from build123d import *

# Parameters (mm, degrees)
F0_R           = 29
F1_DEPTH       = 6
F9_R           = 1.5
F12_DEPTH      = 5
F12_DEPTH_BACK = 10
F10_R          = 1.5
F13_DEPTH      = 5
F13_DEPTH_BACK = 10
F8_R           = 1.5
F14_DEPTH      = 5
F14_DEPTH_BACK = 10
F11_R          = 1.5
F15_DEPTH      = 5
F15_DEPTH_BACK = 10
F4_R           = 1.5
F16_DEPTH      = 5
F16_DEPTH_BACK = 10
F7_R           = 1.5
F17_DEPTH      = 5
F17_DEPTH_BACK = 10
F6_R           = 1.5
F18_DEPTH      = 5
F18_DEPTH_BACK = 10
F5_R           = 1.5
F19_DEPTH      = 5
F19_DEPTH_BACK = 10
F3_R           = 1.5
F20_DEPTH      = 5
F20_DEPTH_BACK = 10
F21_R          = 36.5
F21_R_2        = 31.775
F22_DEPTH      = 6
F2_R           = 1.5
F23_DEPTH      = 10


with BuildPart() as f1:
    # F0 (on Top) → F1 (new body)
    with BuildSketch(Plane.XY):
        Polygon((33.286979, -10.815593), (33.286977, 10.815597), (20.572482, 28.315596), (-2e-06, 35), (-20.572485, 28.315594), (-33.286979, 10.815593), (-33.286977, -10.815597), (-20.572482, -28.315596), (2e-06, -35), (20.572485, -28.315594), align=None)
        Circle(F0_R, mode=Mode.SUBTRACT)
    extrude(amount=F1_DEPTH)

    # F9 (on face) → F12 (cut, two sides)
    with BuildSketch(Plane(origin=(-33.286978, -2e-06, 0), x_dir=(0, -1, 0), z_dir=(-1, 0, 0))) as f12_sk:
        with Locations((0.000595, 3)):
            Circle(F9_R)
    extrude(amount=-F12_DEPTH, mode=Mode.SUBTRACT)
    extrude(f12_sk.sketch, amount=-F12_DEPTH_BACK, mode=Mode.SUBTRACT)

    # F10 (on face) → F13 (cut, two sides)
    with BuildSketch(Plane(origin=(10.286244, -31.657797, 0), x_dir=(0.951056, 0.309017, 0), z_dir=(0.309017, -0.951056, 0))) as f13_sk:
        with Locations((-1.499405, 3)):
            Circle(F10_R)
    extrude(amount=-F13_DEPTH, mode=Mode.SUBTRACT)
    extrude(f13_sk.sketch, amount=-F13_DEPTH_BACK, mode=Mode.SUBTRACT)

    # F8 (on face) → F14 (cut, two sides)
    with BuildSketch(Plane(origin=(33.286978, 2e-06, 0), x_dir=(0, 1, 0), z_dir=(1, 0, 0))) as f14_sk:
        with Locations((0.000595, 3)):
            Circle(F8_R)
    extrude(amount=F14_DEPTH, mode=Mode.SUBTRACT)
    extrude(f14_sk.sketch, amount=-F14_DEPTH_BACK, mode=Mode.SUBTRACT)

    # F11 (on face) → F15 (cut, two sides)
    with BuildSketch(Plane(origin=(26.929732, -19.565593, 0), x_dir=(0.587785, 0.809017, 0), z_dir=(0.809017, -0.587785, 0))) as f15_sk:
        with Locations((-1.499405, 3)):
            Circle(F11_R)
    extrude(amount=F15_DEPTH, mode=Mode.SUBTRACT)
    extrude(f15_sk.sketch, amount=-F15_DEPTH_BACK, mode=Mode.SUBTRACT)

    # F4 (on face) → F16 (cut, two sides)
    with BuildSketch(Plane(origin=(-26.92973, -19.565596, 0), x_dir=(0.587785, -0.809017, 0), z_dir=(-0.809017, -0.587785, 0))) as f16_sk:
        with Locations((0.000595, 3)):
            Circle(F4_R)
    extrude(amount=F16_DEPTH, mode=Mode.SUBTRACT)
    extrude(f16_sk.sketch, amount=-F16_DEPTH_BACK, mode=Mode.SUBTRACT)

    # F7 (on face) → F17 (cut, two sides)
    with BuildSketch(Plane(origin=(-26.929732, 19.565593, 0), x_dir=(-0.587785, -0.809017, 0), z_dir=(-0.809017, 0.587785, 0))) as f17_sk:
        with Locations((0.000595, 3)):
            Circle(F7_R)
    extrude(amount=F17_DEPTH, mode=Mode.SUBTRACT)
    extrude(f17_sk.sketch, amount=-F17_DEPTH_BACK, mode=Mode.SUBTRACT)

    # F6 (on face) → F18 (cut, two sides)
    with BuildSketch(Plane(origin=(26.92973, 19.565596, 0), x_dir=(-0.587785, 0.809017, 0), z_dir=(0.809017, 0.587785, 0))) as f18_sk:
        with Locations((0.000595, 3)):
            Circle(F6_R)
    extrude(amount=-F18_DEPTH, mode=Mode.SUBTRACT)
    extrude(f18_sk.sketch, amount=-F18_DEPTH_BACK, mode=Mode.SUBTRACT)

    # F5 (on face) → F19 (cut, two sides)
    with BuildSketch(Plane(origin=(-10.28624, -31.657798, 0), x_dir=(0.951057, -0.309017, 0), z_dir=(-0.309017, -0.951057, 0))) as f19_sk:
        with Locations((0.000595, 3)):
            Circle(F5_R)
    extrude(amount=-F19_DEPTH, mode=Mode.SUBTRACT)
    extrude(f19_sk.sketch, amount=-F19_DEPTH_BACK, mode=Mode.SUBTRACT)

    # F3 (on face) → F20 (cut, two sides)
    with BuildSketch(Plane(origin=(10.28624, 31.657798, 0), x_dir=(-0.951057, 0.309017, 0), z_dir=(0.309017, 0.951057, 0))) as f20_sk:
        with Locations((0.000595, 3)):
            Circle(F3_R)
    extrude(amount=-F20_DEPTH, mode=Mode.SUBTRACT)
    extrude(f20_sk.sketch, amount=-F20_DEPTH_BACK, mode=Mode.SUBTRACT)

    # F21 (on Top) → F22 (cut)
    with BuildSketch(Plane.XY):
        Circle(F21_R)
        Circle(F21_R_2, mode=Mode.SUBTRACT)
    extrude(amount=F22_DEPTH, mode=Mode.SUBTRACT)

    # F2 (on face) → F23 (cut)
    with BuildSketch(Plane(origin=(-10.286244, 31.657797, 0), x_dir=(-0.951056, -0.309017, 0), z_dir=(-0.309017, 0.951056, 0))):
        with Locations((0.000595, 3)):
            Circle(F2_R)
    extrude(amount=-F23_DEPTH, mode=Mode.SUBTRACT)


solid = f1.part
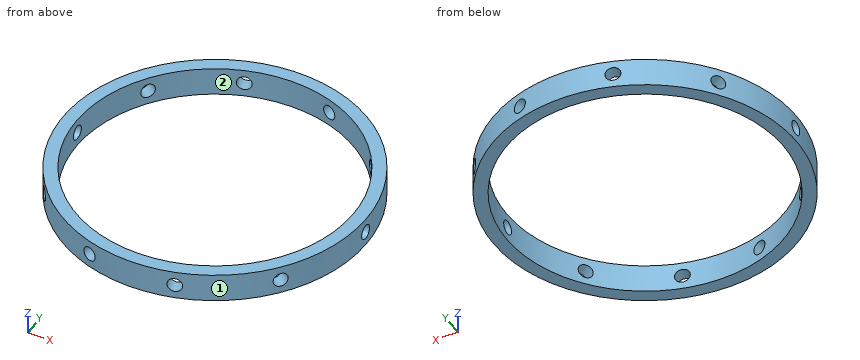
CAD build for the part. Positions are in the model's coordinates, mm. Face numbers are marked on the shaded views. Give positions to 0.01 mm unless a question says otherwise; leave off trailing zeros. Write each loop counter-clockwise with the first axis right and the second up, starting at its lowest first coordinate (ties: lowest second). Pieces come first, ordered by that corner, then holes. Notation, with made-up numbers: (89.25, 29) - (99.25, 29) arc R15 cw to (99.25, 53) - close; hole circle Ø1 at (-6.75, 86). An arc over 180 degrees is marked (long way). Put each result on its own line as item: value.
(1) Pull direction Y, two halves, no side cores. Call the marked faces 1 and 2: released by +Y, released by -Y, zero draft, split by the parting line, or undercut.
Working result:
face 1: split by the parting line
face 2: undercut
(2) Saw through at D-D (z = 2.25). Count the separate pieces of the cut face and the enclosed holes in it, then the cut area to 3 significant figures.
Working result:
separate pieces: 10
enclosed holes: 0
area: 458 mm^2
(3) Wall check: L1, parallel to Y at x = 0, z = 2.25 (3 decimals); L2, parallel to X at y = 24.5, z = 3.25; L3, parallel to X at y = 25, z = 2.25. Give the ranges that are in metal, low to high.
Working result:
L1: -31.775 to -29, 29 to 31.775
L2: -20.23 to -15.52, 15.52 to 20.23
L3: -19.61 to -14.7, 14.7 to 19.61
(4) Saw through at C-C (y = 23.5). List the corners of the cut face in (x, z), then the cut area to 3 significant figures.
Working result:
outline: (-21.39, 0) - (-16.99, 0) - (-16.99, 6) - (-21.39, 6) - close; (16.99, 0) - (21.39, 0) - (21.39, 6) - (16.99, 6) - close
area: 52.7 mm^2
(5) Saw through at B-B (x = 0). List the corners of the cut face in (y, z) (3 decimals).
Working result:
outline: (-31.775, 0) - (-29, 0) - (-29, 6) - (-31.775, 6) - close; (29, 0) - (31.775, 0) - (31.775, 6) - (29, 6) - close
(6) Drop flat-ended pins along their axis: pin 1 Ø1 at (x, z) = (-17.5, 1) entering from -Y; pin 2 Ø3.5 at (y, z) = (0, 3) entering from +X (3 decimals). Give the stop position or say it passes through.
Working result:
pin 1: y = -26.84
pin 2: x = 31.775
(7) Saw through at A-A (y = 0). List the corners of the cut face in (x, z) (3 decimals).
Working result:
outline: (-31.775, 0) - (-29, 0) - (-29, 1.5) - (-31.775, 1.5) - close; (-31.775, 4.5) - (-29, 4.5) - (-29, 6) - (-31.775, 6) - close; (29, 0) - (31.775, 0) - (31.775, 1.5) - (29, 1.5) - close; (29, 4.5) - (31.775, 4.5) - (31.775, 6) - (29, 6) - close
